Autodesk Inventor part; units mm, degrees
ref_plane "YZ Plane" through (0, 0, 0) normal (1, 0, 0) x (0, 1, 0)
ref_plane "XZ Plane" through (0, 0, 0) normal (0, 1, 0) x (-1, 0, 0)
ref_plane "XY Plane" through (0, 0, 0) normal (0, 0, 1) x (1, 0, 0)
sketch "Sketch1" plane through (0, 0, 0) normal (0, 1, 0) x (-1, 0, 0)
  line L0 (-177.8, 114.3) -> (177.8, 114.3)
  line L1 (177.8, 114.3) -> (177.8, -114.3)
  line L2 (177.8, -114.3) -> (-177.8, -114.3)
  line L3 (-177.8, -114.3) -> (-177.8, 114.3)
  line L4 (-177.8, 114.3) -> (177.8, -114.3) construction
  line L5 (177.8, 114.3) -> (-177.8, -114.3) construction
  line L6 (-165.1, 95.25) -> (-177.8, 95.25)
  line L7 (-177.8, 95.25) -> (-177.8, 3.81)
  line L8 (-177.8, 3.81) -> (-165.1, 3.81)
  line L9 (-165.1, 3.81) -> (-165.1, 95.25)
  line L10 (-165.1, -3.81) -> (-177.8, -3.81)
  line L11 (-177.8, -3.81) -> (-177.8, -95.25)
  line L12 (-177.8, -95.25) -> (-165.1, -95.25)
  line L13 (-165.1, -95.25) -> (-165.1, -3.81)
  line L14 (-146.05, 72.39) -> (-146.05, 26.67) construction
  line L15 (-149.86, 72.39) -> (-149.86, 26.67)
  line L16 (-142.24, 26.67) -> (-142.24, 72.39)
  arc A0 (-142.24, 72.39) -> (-149.86, 72.39) centre (-146.05, 72.39) ccw
  arc A1 (-149.86, 26.67) -> (-142.24, 26.67) centre (-146.05, 26.67) ccw
  line L17 (-146.05, -26.67) -> (-146.05, -72.39) construction
  line L18 (-149.86, -26.67) -> (-149.86, -72.39)
  line L19 (-142.24, -72.39) -> (-142.24, -26.67)
  arc A2 (-142.24, -26.67) -> (-149.86, -26.67) centre (-146.05, -26.67) ccw
  arc A3 (-149.86, -72.39) -> (-142.24, -72.39) centre (-146.05, -72.39) ccw
  point P0 (0, 0)
  point P1 (-146.05, 49.53)
  point P2 (-146.05, -49.53)
  point P3 (-177.8, 3.81)
  dimension "d0" = 355.6
  dimension "d1" = 228.6
  dimension "d2" = 12.7
  dimension "d3" = 91.44
  dimension "d4" = 91.44
  dimension "d5" = 12.7
  dimension "d6" = 19.05
  dimension "d7" = 19.05
  dimension "d8" = 45.72
  dimension "d9" = 7.62
  dimension "d10" = 45.72
  dimension "d11" = 7.62
  dimension "d12" = 41.91
  dimension "d13" = 19.05
  dimension "d14" = 19.05
  dimension "d15" = 41.91
extrude "Extrusion1" add sketch "Sketch1" along normal blind 1.5875 contours L0 L1 L2 L3 L12 L13 L10 L8 L9 L6
properties part number "EBox Door" material "Aluminum 6061"
Geometry check sheet. Reference: the model listing, model coordinates, mm. Coordinates: 2 decimals unless noted, no trailing zeros. Loops run counter-clockwise (first coordinate to the right, second up) from the corner with the lowest first, then second, coordinate; pieces in that order, holes last. Notation, with made-up numbers: (61.5, 75) - (84.5, 75) arc R35 ccw to (84.5, 108) - close; hole circle Ø4 at (74, 32). An arc over 180 degrees is marked (long way). Use one line per item in the form item = value. Start each with the question number.
Item 1: Gauge pin test, flat end, axial feed: pin 1 (0.5 mm diameter, centred on y = 0.5, z = 41.5, fed in from +X). Record the tip position at first contact, or that the pin passes through.
Item 2: Section check C-C, the plane z = -66.5. Enter the section's corners in (x, y), and give its area (3 significant figures).
Item 3: Section check B-B, the plane y = 0.6. Enter the section's corners in (x, z), and give its area (3 significant figures).
Item 4: Section check D-D, the plane z = -9.5. Enter the section's corners in (x, y), and give its area (3 significant figures).
Item 5: Thickness scan on probe 1 along X at (y, z) = (0.4, 51.5); probe 2 along X at (y, z) = (0.7, 4). Record the ranges inside material, lowest first.
Item 6: Section check A-A, the plane x = 146.05. Enter the section's corners in (y, z).
Computed:
q1.pin_1 = 165.1
q2.outline = (-177.8, 0) - (142.24, 0) - (142.24, 1.59) - (-177.8, 1.59) - close; (149.86, 0) - (165.1, 0) - (165.1, 1.59) - (149.86, 1.59) - close
q2.area = 532 mm2
q3.outline = (-177.8, -114.3) - (177.8, -114.3) - (177.8, -95.25) - (165.1, -95.25) - (165.1, -3.81) - (177.8, -3.81) - (177.8, 3.81) - (165.1, 3.81) - (165.1, 95.25) - (177.8, 95.25) - (177.8, 114.3) - (-177.8, 114.3) - close; hole (142.24, -72.39) arc R3.81 ccw to (149.86, -72.39) - (149.86, -26.67) arc R3.81 ccw to (142.24, -26.67) - close; hole (142.24, 26.67) arc R3.81 ccw to (149.86, 26.67) - (149.86, 72.39) arc R3.81 ccw to (142.24, 72.39) - close
q3.area = 78,200 mm2
q4.outline = (-177.8, 0) - (165.1, 0) - (165.1, 1.59) - (-177.8, 1.59) - close
q4.area = 544 mm2
q5.probe_1 = -177.8 to 142.24, 149.86 to 165.1
q5.probe_2 = -177.8 to 165.1
q6.outline = (0, -114.3) - (1.59, -114.3) - (1.59, -76.2) - (0, -76.2) - close; (0, -22.86) - (1.59, -22.86) - (1.59, 22.86) - (0, 22.86) - close; (0, 76.2) - (1.59, 76.2) - (1.59, 114.3) - (0, 114.3) - close
